from build123d import *

# Parameters (mm, degrees)
F0_W     = 65.000124
F0_H     = 5.08
F1_DEPTH = 25.4
F2_SIZE2 = 4.6224219752
F2_SIZE  = 12.7
F3_R     = 5.07999


# Not quite as in the source:
# - a fillet or chamfer is up to 0.001 mm smaller than in the source, because OpenCascade refuses the exact size


with BuildPart() as f1:
    # F0 (on Top) → F1 (new body)
    with BuildSketch(Plane.XY):
        with Locations((-11.0949875303, 2.54)):
            Rectangle(F0_W, F0_H)
    extrude(amount=F1_DEPTH)

    # F2
    f2_edges = [f1.edges().sort_by_distance(p)[0] for p in [
        (-11.094988, 5.08, 25.4),
    ]]
    f2_side = f1.faces().sort_by_distance((-11.094988, 5.08, 12.7))[0]
    chamfer(f2_edges, length=F2_SIZE, length2=F2_SIZE2, reference=f2_side)

    # F3 (radius 5.08 in the source; OpenCascade refuses exactly that, so slightly less here)
    f3_edges = [f1.edges().sort_by_distance(p)[0] for p in [
        (21.405074, 2.768789, 19.05),
        (21.405074, 5.08, 6.35),
        (-43.59505, 5.08, 6.35),
        (-43.59505, 2.768789, 19.05),
    ]]
    fillet(f3_edges, radius=F3_R)


solid = f1.part
Check sheet for the modelled part. Datum: model origin and axes. Units: mm. Give positions to 0.01 mm unless a question says otherwise; leave off trailing zeros. Order: outer loops, then holes, each group sorted by start corner. A loop starts at its lowest first (then second) coordinate and runs counter-clockwise, first axis right, second up. Notation, with made-up numbers: (16.25, -29) - (54.25, -29) arc R24 ccw to (54.25, -4) - close; hole circle Ø4 at (-8.75, 71.25). An arc over 180 degrees is marked (long way). Answer as CSV lines item,"result".
1. Scan lines: probe 1 along X at (y, z) = (4.65, 3); probe 2 along Y at (x, z) = (-36, 17.5); probe 3 along X at (y, z) = (2.4, 3.5). Record each from-to range of solid material in increasing order. Write a range as from..to.
Result sheet:
probe 1,"-40.56..18.37"
probe 2,"0..3.33"
probe 3,"-42.99..20.8"
2. Go/stop test with flat-tipped pins: P1, Ø5, axis at x = -17.5, z = 22, coming from the +Y side (3 decimals); P2, Ø1.5, axis at x = -17.5, z = 19.5, coming from the +Y side. Record where each tip stops, or that it passes through.
Result sheet:
P1,"y = 2.605"
P2,"y = 2.88"
3. Section check B-B (x = -32). Record the boundary of the cut face in (y, z).
Result sheet:
outline,"(0, 0) - (5.08, 0) - (5.08, 12.7) - (0.46, 25.4) - (0, 25.4) - close"
